The model under review builds one solid part; all positions refer to its coordinate system, in mm. A direction names the side the tool comes from. Give positions to 0.01 mm unless a question says otherwise; leave off trailing zeros. Order: outer loops, then holes, each group sorted by start corner. A loop starts at its lowest first (then second) coordinate and runs counter-clockwise, first axis right, second up.
Autodesk Inventor part; units mm, degrees
ref_plane "YZ Plane" through (0, 0, 0) normal (1, 0, 0) x (0, 1, 0)
ref_plane "XZ Plane" through (0, 0, 0) normal (0, 1, 0) x (-1, 0, 0)
ref_plane "XY Plane" through (0, 0, 0) normal (0, 0, 1) x (1, 0, 0)
sketch "Sketch3" plane through (0, 0, 0) normal (1, 0, 0) x (0, 1, 0)
  circle A0 centre (0, 0) radius 11.7
  dimension "d1" = 23.4
extrude "Extrusion1" add sketch "Sketch3" along normal mid plane 90
sketch "Sketch4" plane through (45, 0, 0) normal (1, 0, 0) x (0, 0, -1)
  point P0 (0, 0)
sketch "Sketch5" plane through (-45, 0, 0) normal (-1, 0, 0) x (0, 0, 1)
  circle A0 centre (0, 0) radius 11.7
  circle A1 centre (0, 0) radius 50
  dimension "d4" = 100
extrude "Extrusion2" add sketch "Sketch5" along normal mid plane 100 contours A0 | A1
sketch "Sketch6" plane through (-95, 0, 0) normal (-1, 0, 0) x (0, 0, 1)
  circle A0 centre (0, 0) radius 11.7
  circle A1 centre (0, 0) radius 43.0072
  circle A2 centre (0, 0) radius 50
extrude "Extrusion3" cut sketch "Sketch6" against normal blind 10 contours A2
fillet "Fillet1" radius 2 1 edges at (-85, 0, -50)
fillet "Fillet2" radius 2 1 edges at (-95, 0, -43.0072)
thread "Thread1"
fillet "Fillet3" radius 2 1 edges at (5, 0, -50)
sketch "Sketch7" plane through (45, 0, 0) normal (1, 0, 0) x (0, 0, -1)
  circle A0 centre (0, 0) radius 23.4
  dimension "d14" = 46.8
extrude "Extrusion4" add sketch "Sketch7" against normal blind 50
properties part number "Motor"
Item 1: Take a section at A-A (z = 0). Give the boundary of the cut face in (x, y), and give its area (3 significant figures).
Values found:
outline: (-95, -41.01) arc R2 ccw to (-93, -43.01) - (-85, -43.01) - (-85, -48) arc R2 ccw to (-83, -50) - (3, -50) arc R2 ccw to (5, -48) - (5, -23.4) - (45, -23.4) - (45, 23.4) - (5, 23.4) - (5, 48) arc R2 ccw to (3, 50) - (-83, 50) arc R2 ccw to (-85, 48) - (-85, 43.01) - (-93, 43.01) arc R2 ccw to (-95, 41.01) - close
area: 11,700 mm2
Item 2: For faces 1 (the flat face through (5, 11, 21)), 2 (the cylindrical face through (-89.06, -26.17, -34.13)), 3 (the flat face through (-95, 1, -1)), list the 3-axis set-ups (+Z, -Z, +X, -X, +Y, -Y) from which the entire face can be reached by the end or side of a thin tool; tool diameter is ignored.
Values found:
face 1: +X
face 2: -X
face 3: +Z, -Z, -X, +Y, -Y
Item 3: For line 1 (X direction, y = 45, z = -10); line 2 (Y direction, x = -72, z = 0); line 3 (X direction, y = 10, z = 26.5), list the stretches that pass through material, from the lowest coordinate up.
Values found:
line 1: x = -85 to 5
line 2: y = -50 to 50
line 3: x = -95 to 5
Item 4: Take a section at C-C (x = -75). Give the boundary of the cut face in (y, z).
Values found:
outline: circle Ø100 at (0, 0)
Item 5: Clearance check with flat-ended pins moving along their axes: pin 1 Ø10 at (x, y) = (-62.5, -4.5) entering from -Z; pin 2 Ø6 at (y, z) = (31.5, -35.5) entering from -X; pin 3 Ø10 at (x, z) = (14, 13) entering from +Y; pin 4 Ø12 at (x, y) = (-43, 22.5) entering from +Z. State where each tip first meets the part, or that it passes through.
Values found:
pin 1: stops at z = -50
pin 2: stops at x = -85
pin 3: stops at y = 21.99
pin 4: stops at z = 47.2
